Source: CAD feature listing. Evaluate the final solid. Frame: model axes, mm. Coordinates: 2 decimals unless noted, no trailing zeros. Order: outer loops, then holes, each group sorted by start corner. A loop starts at its lowest first (then second) coordinate and runs counter-clockwise, first axis right, second up.
```python
from build123d import *

# Parameters (mm, degrees)
BASE_FLANGE1_DEPTH        = 130
UNFOLD1_DEPTH             = 130
UNFOLD1_2_DEPTH           = 130
SKETCH6_W                 = 0.3
SKETCH6_H                 = 8
CUT_EXTRUDE1_DEPTH        = 235.985371885
LPATTERN1_COUNT           = 3
LPATTERN1_PITCH           = 11
LPATTERN2_COUNT           = 3
LPATTERN2_PITCH           = 100
LPATTERN2_COPY_1_SKETCH_W = 0.3
LPATTERN2_COPY_1_SKETCH_H = 8
LPATTERN2_COPY_1_DEPTH    = 235.985371885
LPATTERN2_COPY_2_SKETCH_W = 0.3
LPATTERN2_COPY_2_SKETCH_H = 8
LPATTERN2_COPY_2_DEPTH    = 235.985371885
LPATTERN2_COPY_3_SKETCH_W = 0.3
LPATTERN2_COPY_3_SKETCH_H = 8
LPATTERN2_COPY_3_DEPTH    = 235.985371885
LPATTERN2_COPY_4_SKETCH_W = 0.3
LPATTERN2_COPY_4_SKETCH_H = 8
LPATTERN2_COPY_4_DEPTH    = 235.985371885
FOLD1_DEPTH               = 130
FOLD1_2_DEPTH             = 130
FOLD1_START               = 30
FOLD1_3_DEPTH             = 70
FOLD1_START_2             = 8
FOLD1_4_DEPTH             = 3
FOLD1_START_3             = 19
FOLD1_5_DEPTH             = 3
FOLD1_START_4             = 108
FOLD1_6_DEPTH             = 3
FOLD1_START_5             = 119
FOLD1_7_DEPTH             = 3


# Read off the part's stored shape, not the designer's step: Unfold1, Fold1
# Sheet-metal steps are written as plain solids
with BuildPart() as part:
    # Sketch1 → Base-Flange1 (new body)
    with BuildSketch(Plane(origin=(0, 0, 0), x_dir=(1, 0, 0), z_dir=(0, 1, 0))):
        with BuildLine():
            ThreePointArc((195.5, 0), (195.436009031, 5.001637134), (195.244078015, 10))
            Line((195.244078015, 10), (195.493750749, 10.012787724))
            ThreePointArc((195.493750749, 10.012787724), (195.685927201, 5.008033089), (195.75, 0))
            Line((195.75, 0), (195.5, 0))
        make_face()
    extrude(amount=BASE_FLANGE1_DEPTH)

    # Unfold1 outline → Unfold1 (cut)
    with BuildSketch(Plane(origin=(0, 0, 0), x_dir=(1, 0, 0), z_dir=(0, 1, 0))):
        with BuildLine():
            Line((195.5, 0), (195.5, 9.890020218))
            ThreePointArc((195.5, 9.890020218), (195.496885011, 9.951404462), (195.493750749, 10.012787724))
            Line((195.493750749, 10.012787724), (195.244078015, 10))
            ThreePointArc((195.244078015, 10), (195.436009031, 5.001637134), (195.5, 0))
        make_face()
    extrude(amount=UNFOLD1_DEPTH, mode=Mode.SUBTRACT)

    # Unfold1 2 outline → Unfold1 2 (add)
    with BuildSketch(Plane(origin=(0, 0, 0), x_dir=(1, 0, 0), z_dir=(0, 1, 0))):
        with BuildLine():
            Line((195.75, 0), (195.75, 10.010762486))
            Line((195.75, 10.010762486), (195.5, 10.010762486))
            Line((195.5, 10.010762486), (195.5, 9.890020218))
            ThreePointArc((195.5, 9.890020218), (195.687490019, 4.946589732), (195.75, 0))
        make_face()
    extrude(amount=UNFOLD1_2_DEPTH)

    # Sketch6 → Cut-Extrude1 (cut, symmetric)
    with BuildSketch(Plane(origin=(195.75, 0, -195.75), x_dir=(0, 0, 1), z_dir=(-1, 0, 0))):
        with Locations((185.739237514, 126)):
            Rectangle(SKETCH6_W, SKETCH6_H)
    cut_extrude1 = extrude(amount=CUT_EXTRUDE1_DEPTH, both=True, mode=Mode.SUBTRACT)

    # LPattern1: Cut-Extrude1 ×3
    with Locations(*[(0, -i * LPATTERN1_PITCH, 0) for i in range(1, LPATTERN1_COUNT)]):
        add(cut_extrude1, mode=Mode.SUBTRACT)

    # LPattern2: Cut-Extrude1 ×3
    with Locations(*[(0, -i * LPATTERN2_PITCH, 0) for i in range(1, LPATTERN2_COUNT)]):
        add(cut_extrude1, mode=Mode.SUBTRACT)

    # LPattern2 copy 1 sketch → LPattern2 copy 1 (cut, symmetric)
    with BuildSketch(Plane(origin=(195.75, -111, -195.75), x_dir=(0, 0, 1), z_dir=(-1, 0, 0))):
        with Locations((185.739237514, 126)):
            Rectangle(LPATTERN2_COPY_1_SKETCH_W, LPATTERN2_COPY_1_SKETCH_H)
    extrude(amount=LPATTERN2_COPY_1_DEPTH, both=True, mode=Mode.SUBTRACT)

    # LPattern2 copy 2 sketch → LPattern2 copy 2 (cut, symmetric)
    with BuildSketch(Plane(origin=(195.75, -211, -195.75), x_dir=(0, 0, 1), z_dir=(-1, 0, 0))):
        with Locations((185.739237514, 126)):
            Rectangle(LPATTERN2_COPY_2_SKETCH_W, LPATTERN2_COPY_2_SKETCH_H)
    extrude(amount=LPATTERN2_COPY_2_DEPTH, both=True, mode=Mode.SUBTRACT)

    # LPattern2 copy 3 sketch → LPattern2 copy 3 (cut, symmetric)
    with BuildSketch(Plane(origin=(195.75, -122, -195.75), x_dir=(0, 0, 1), z_dir=(-1, 0, 0))):
        with Locations((185.739237514, 126)):
            Rectangle(LPATTERN2_COPY_3_SKETCH_W, LPATTERN2_COPY_3_SKETCH_H)
    extrude(amount=LPATTERN2_COPY_3_DEPTH, both=True, mode=Mode.SUBTRACT)

    # LPattern2 copy 4 sketch → LPattern2 copy 4 (cut, symmetric)
    with BuildSketch(Plane(origin=(195.75, -222, -195.75), x_dir=(0, 0, 1), z_dir=(-1, 0, 0))):
        with Locations((185.739237514, 126)):
            Rectangle(LPATTERN2_COPY_4_SKETCH_W, LPATTERN2_COPY_4_SKETCH_H)
    extrude(amount=LPATTERN2_COPY_4_DEPTH, both=True, mode=Mode.SUBTRACT)

    # Fold1 outline → Fold1 (cut)
    with BuildSketch(Plane(origin=(0, 0, 0), x_dir=(1, 0, 0), z_dir=(0, 1, 0))):
        with BuildLine():
            ThreePointArc((195.5, 9.890020218), (195.687490019, 4.946589732), (195.75, 0))
            Line((195.75, 0), (195.75, 10.010762486))
            Line((195.75, 10.010762486), (195.5, 10.010762486))
            Line((195.5, 10.010762486), (195.5, 9.890020218))
        make_face()
    extrude(amount=FOLD1_DEPTH, mode=Mode.SUBTRACT)

    # Fold1 2 outline → Fold1 2 (add)
    with BuildSketch(Plane(origin=(0, 0, 0), x_dir=(1, 0, 0), z_dir=(0, 1, 0))):
        with BuildLine():
            ThreePointArc((195.25168835, 9.850289156), (195.437912228, 4.926709225), (195.5, 0))
            Line((195.5, 0), (195.5, 9.860762486))
            Line((195.5, 9.860762486), (195.501477905, 9.860762486))
            ThreePointArc((195.501477905, 9.860762486), (195.501424363, 9.86182396), (195.501370816, 9.862885433))
            Line((195.501370816, 9.862885433), (195.25168835, 9.850289156))
        make_face()
    extrude(amount=FOLD1_2_DEPTH)

    # Fold1 3 outline → Fold1 3 (add)
    with BuildSketch(Plane(origin=(0, 0, 0), x_dir=(1, 0, 0), z_dir=(0, 1, 0)).offset(FOLD1_START)):
        with BuildLine():
            ThreePointArc((195.244078015, 10), (195.247897532, 9.925145307), (195.25168835, 9.850289156))
            Line((195.25168835, 9.850289156), (195.5, 9.862816276))
            Line((195.5, 9.862816276), (195.5, 9.890020218))
            ThreePointArc((195.5, 9.890020218), (195.496885011, 9.951404462), (195.493750749, 10.012787724))
            Line((195.493750749, 10.012787724), (195.244078015, 10))
        make_face()
    extrude(amount=FOLD1_3_DEPTH)

    # Fold1 4 outline → Fold1 4 (add)
    with BuildSketch(Plane(origin=(0, 0, 0), x_dir=(1, 0, 0), z_dir=(0, 1, 0)).offset(FOLD1_START_2)):
        with BuildLine():
            ThreePointArc((195.244078015, 10), (195.247897532, 9.925145307), (195.25168835, 9.850289156))
            Line((195.25168835, 9.850289156), (195.5, 9.862816276))
            Line((195.5, 9.862816276), (195.5, 9.890020218))
            ThreePointArc((195.5, 9.890020218), (195.496885011, 9.951404462), (195.493750749, 10.012787724))
            Line((195.493750749, 10.012787724), (195.244078015, 10))
        make_face()
    extrude(amount=FOLD1_4_DEPTH)

    # Fold1 5 outline → Fold1 5 (add)
    with BuildSketch(Plane(origin=(0, 0, 0), x_dir=(1, 0, 0), z_dir=(0, 1, 0)).offset(FOLD1_START_3)):
        with BuildLine():
            ThreePointArc((195.244078015, 10), (195.247897532, 9.925145307), (195.25168835, 9.850289156))
            Line((195.25168835, 9.850289156), (195.5, 9.862816276))
            Line((195.5, 9.862816276), (195.5, 9.890020218))
            ThreePointArc((195.5, 9.890020218), (195.496885011, 9.951404462), (195.493750749, 10.012787724))
            Line((195.493750749, 10.012787724), (195.244078015, 10))
        make_face()
    extrude(amount=FOLD1_5_DEPTH)

    # Fold1 6 outline → Fold1 6 (add)
    with BuildSketch(Plane(origin=(0, 0, 0), x_dir=(1, 0, 0), z_dir=(0, 1, 0)).offset(FOLD1_START_4)):
        with BuildLine():
            ThreePointArc((195.244078015, 10), (195.247897532, 9.925145307), (195.25168835, 9.850289156))
            Line((195.25168835, 9.850289156), (195.5, 9.862816276))
            Line((195.5, 9.862816276), (195.5, 9.890020218))
            ThreePointArc((195.5, 9.890020218), (195.496885011, 9.951404462), (195.493750749, 10.012787724))
            Line((195.493750749, 10.012787724), (195.244078015, 10))
        make_face()
    extrude(amount=FOLD1_6_DEPTH)

    # Fold1 7 outline → Fold1 7 (add)
    with BuildSketch(Plane(origin=(0, 0, 0), x_dir=(1, 0, 0), z_dir=(0, 1, 0)).offset(FOLD1_START_5)):
        with BuildLine():
            ThreePointArc((195.244078015, 10), (195.247897532, 9.925145307), (195.25168835, 9.850289156))
            Line((195.25168835, 9.850289156), (195.5, 9.862816276))
            Line((195.5, 9.862816276), (195.5, 9.890020218))
            ThreePointArc((195.5, 9.890020218), (195.496885011, 9.951404462), (195.493750749, 10.012787724))
            Line((195.493750749, 10.012787724), (195.244078015, 10))
        make_face()
    extrude(amount=FOLD1_7_DEPTH)


solid = part.part
```
1. Section query C-C on z = -7.75. Return loops of the section in (x, y).
Findings:
outline: (195.35, 0) - (195.6, 0) - (195.6, 130) - (195.35, 130) - close
2. Ray query, line 1 (X direction, y = 101, z = -1); line 2 (X direction, y = 67, z = -9.25). Return the intervals inside material, ascending.
Findings:
line 1: x = 195.5 to 195.75
line 2: x = 195.28 to 195.53
3. Pin query (flat end, axial travel): P1, Ø4, axis at y = 78.5, z = -4.5, coming from the +X side; P2, Ø1.5, axis at y = 113.5, z = -4, coming from the -X side. Return the tip coordinate at first contact, or that it passes through.
Findings:
P1: stops at x = 195.73
P2: stops at x = 195.44
